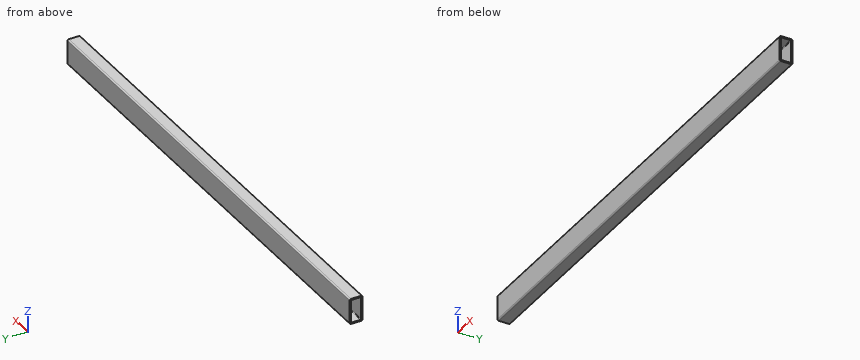
from build123d import *

# Parameters (mm, degrees)
F0_W     = 977.9
F0_H     = 50.8
F1_DEPTH = 12.7
F2_T     = -2.54
F3_R     = 2.54
F4_R     = 1.27


with BuildPart() as f1:
    # F0 (on Front) → F1 (new body, symmetric)
    with BuildSketch(Plane.XZ):
        Rectangle(F0_W, F0_H)
    extrude(amount=F1_DEPTH, both=True)

    # F2
    f2_openings = [f1.faces().sort_by_distance(p)[0] for p in [
        (-488.95, 0, 0),
        (488.95, 0, 0),
    ]]
    offset(amount=F2_T, openings=f2_openings)

    # F3
    f3_edges = [f1.edges().sort_by_distance(p)[0] for p in [
        (0, -12.7, 25.4),
        (0, 12.7, 25.4),
        (0, 12.7, -25.4),
        (0, -12.7, -25.4),
    ]]
    fillet(f3_edges, radius=F3_R)

    # F4
    f4_edges = [f1.edges().sort_by_distance(p)[0] for p in [
        (0, -10.16, 22.86),
        (0, 10.16, 22.86),
        (0, 10.16, -22.86),
        (0, -10.16, -22.86),
    ]]
    fillet(f4_edges, radius=F4_R)


solid = f1.part
Work out the finished part from the listing and answer in its coordinate system (mm). Round coordinates to 2 decimals unless told otherwise and drop trailing zeros. Write each loop counter-clockwise with the first axis right and the second up, starting at its lowest first coordinate (ties: lowest second). Pieces come first, ordered by that corner, then holes. Notation, with made-up numbers: (83.25, 64) - (138.25, 64) arc R6 ccw to (138.25, 68) - close; hole circle Ø6 at (39, 86.5). An arc over 180 degrees is marked (long way). Answer in a Markdown table with one row per item. Add a question column.
1. A cutting plane is placed at C-C, the plane x = 168. Determine the outline of the cut face in (y, z), and give its area (3 significant figures).
2. A cutting plane is placed at A-A, the plane z = -8.5. Determine the outline of the cut face in (x, y).
3. Find the intervals of material crossed by line 1 along Y through (x, z) = (-108, -20); line 2 along Z through (x, y) = (-428, -9); line 3 along Y through (x, z) = (-152, -22), in increasing order. Write a range as from..to.
4. Given pin 1 (3 mm diameter, centred on y = -8, z = 6.5, fed in from +X), flat-ended and moving along its own axis, determine where the tip first touches the part or whether it passes through.
5. A cutting plane is placed at B-B, the plane y = -2.25. Determine the outline of the cut face in (x, z), and give its area (3 significant figures).
Worked out:
| question | item | result |
|---|---|---|
| 1 | outline | (-12.7, -22.86) arc R2.54 ccw to (-10.16, -25.4) - (10.16, -25.4) arc R2.54 ccw to (12.7, -22.86) - (12.7, 22.86) arc R2.54 ccw to (10.16, 25.4) - (-10.16, 25.4) arc R2.54 ccw to (-12.7, 22.86) - close; hole (-10.16, -21.59) arc R1.27 ccw to (-8.89, -22.86) - (8.89, -22.86) arc R1.27 ccw to (10.16, -21.59) - (10.16, 21.59) arc R1.27 ccw to (8.89, 22.86) - (-8.89, 22.86) arc R1.27 ccw to (-10.16, 21.59) - close |
| 1 | area | 357 mm^2 |
| 2 | outline | (-488.95, -12.7) - (488.95, -12.7) - (488.95, -10.16) - (-488.95, -10.16) - close; (-488.95, 10.16) - (488.95, 10.16) - (488.95, 12.7) - (-488.95, 12.7) - close |
| 3 | line 1 | -12.7..-10.16, 10.16..12.7 |
| 3 | line 2 | -25.4..-22.86, 22.86..25.4 |
| 3 | line 3 | -12.7..-10.09, 10.09..12.7 |
| 4 | pin 1 | through |
| 5 | outline | (-488.95, -25.4) - (488.95, -25.4) - (488.95, -22.86) - (-488.95, -22.86) - close; (-488.95, 22.86) - (488.95, 22.86) - (488.95, 25.4) - (-488.95, 25.4) - close |
| 5 | area | 4,970 mm^2 |
